For this review, use the dimensioned drawing (mm, ordinates from the lowest corner) and the shaded views. A direction names the side the tool comes from. Coordinates: 2 decimals unless noted, no trailing zeros. Write each loop counter-clockwise with the first axis right and the second up, starting at its lowest first coordinate (ties: lowest second). Pieces come first, ordered by that corner, then holes.
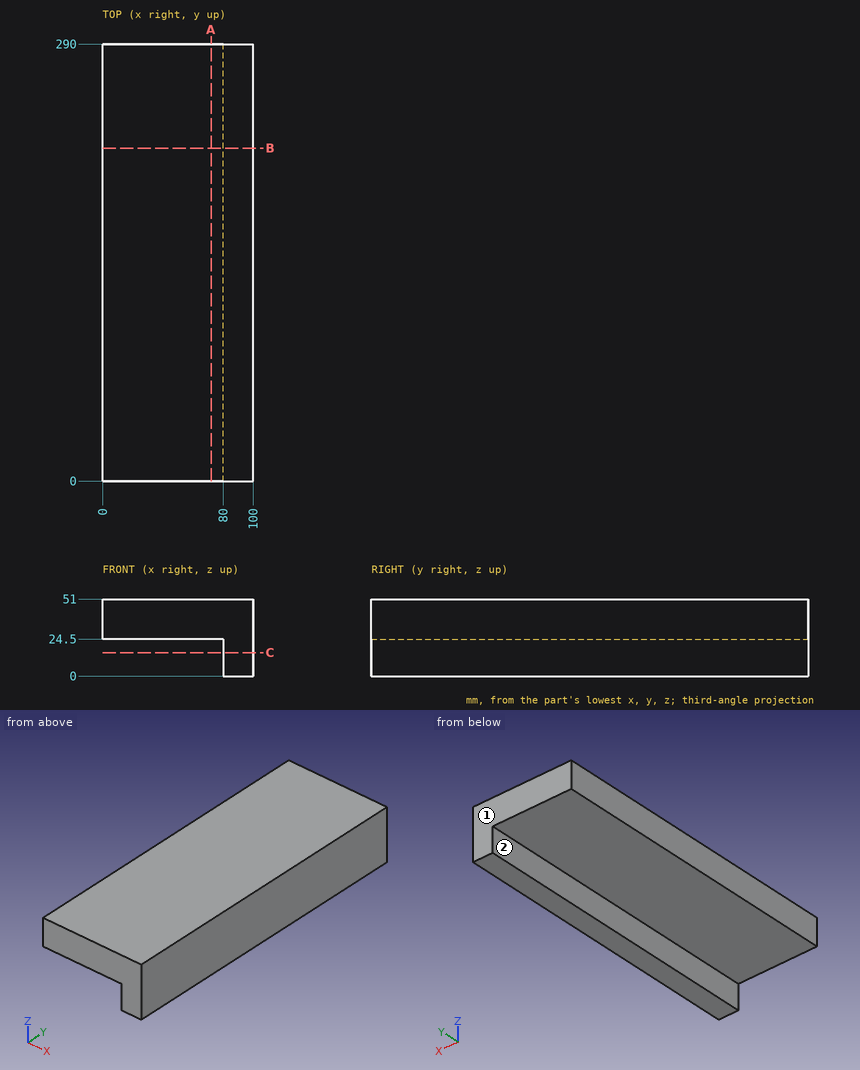
(1) Consider section C-C (z = 15.5). Give the boundary of the cut face in (x, y), plus the area to 3 significant figures.
(2) Consider section B-B (y = 221). Give the boundary of the cut face in (x, z).
(3) Consider section A-A (x = 72). Give the boundary of the cut face in (y, z).
(4) Insertion check: pin 1 Ø19.5 at (y, z) = (171, 14) entering from -X; pin 2 Ø3 at (x, y) = (43.5, 180) entering from -Z. Each pin has a flat end and moves straight along its axis. Give the tip position at first contact, or say it passes through.
(5) Wall thickness on line 1 (Z direction, x = 29.5, y = 227.5); line 2 (X direction, y = 121, z = 18.5): over which ranges is each line inside the solid? List them lowest first.
(6) For the marked faces 1 and 2, list the 3-axis set-ups (+Z, -Z, +X, -X, +Y, -Y) from which the entire face can be reached by the end or side of a thin tool; tool diameter is ignored.
Results:
1. outline: (80, 0) - (100, 0) - (100, 290) - (80, 290) - close
1. area: 5,800 mm2
2. outline: (0, 24.5) - (80, 24.5) - (80, 0) - (100, 0) - (100, 51) - (0, 51) - close
3. outline: (0, 24.5) - (290, 24.5) - (290, 51) - (0, 51) - close
4. pin 1: stops at x = 80
4. pin 2: stops at z = 24.5
5. line 1: z = 24.5 to 51
5. line 2: x = 80 to 100
6. face 1: +Z, -Z, +X, -X, +Y
6. face 2: -Z, -X, +Y, -Y
